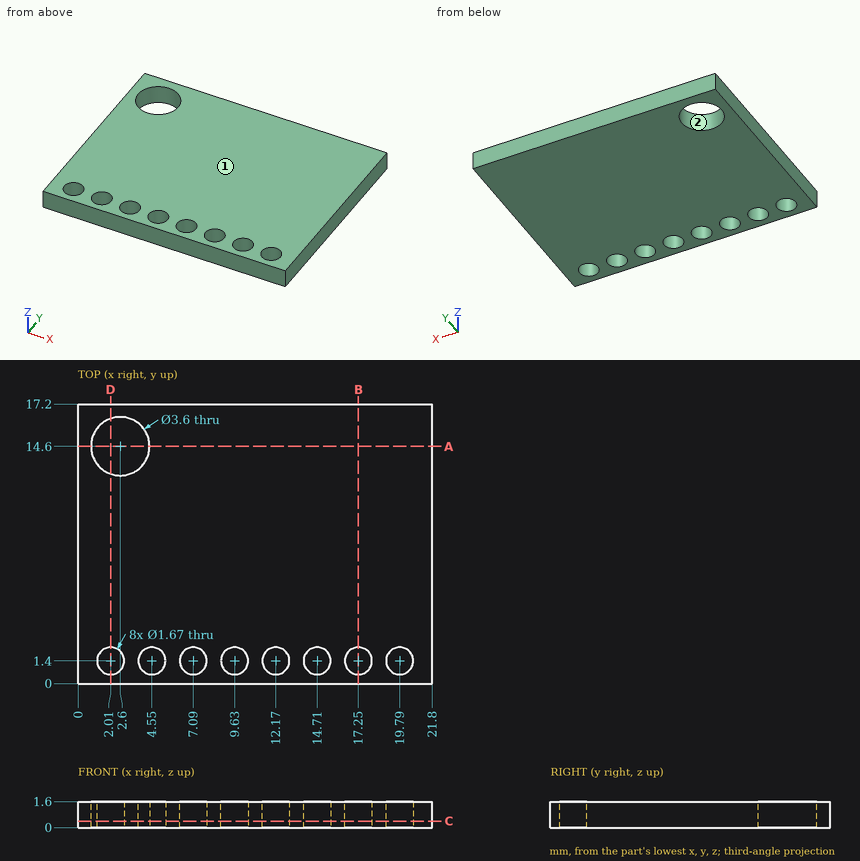
Source: three-view drawing plus pictorial views. Frame: mm from the lowest corner of the part. Round coordinates to 2 decimals unless told otherwise and drop trailing zeros. Loops run counter-clockwise (first coordinate to the right, second up) from the corner with the lowest first, then second, coordinate; pieces in that order, holes last.
1. Contact query for a flat-ended pin moving along its axis: pin 1 (6 mm diameter, centred on x = 10.5, y = 11.5, fed in from -Z). Output: stop coordinate, or through.
2. Section query C-C on z = 0.4. Give the number of separate pieces and of enclosed holes in the cut face, and give its area (3 significant figures).
3. Section query D-D on x = 2.01. Output: boundary loops of the cut face in (y, z) (3 decimals), and give its area (3 significant figures).
4. Section query B-B on x = 17.25. Output: boundary loops of the cut face in (y, z) (3 decimals).
5. Section query A-A on y = 14.6. Output: boundary loops of the cut face in (x, z), and give its area (3 significant figures).
6. Mould query, pull axis Y, two halves, no side actions, for the marked faces 1 and 2. Classes: released by +Y, released by -Y, zero draft, split by the parting line, or undercut.
7. Ray query, L1, parallel to Y at x = 19.79, z = 1.3 (3 decimals); L2, parallel to Y at x = 1.75, z = 0.3; L3, parallel to Y at x = 3.25, z = 0.9. Return the intervals inside material, ascending.
Answers below:
1. pin 1: stops at z = 0
2. separate pieces: 1
2. enclosed holes: 9
2. area: 347 mm2
3. outline: (0, 0) - (0.565, 0) - (0.565, 1.6) - (0, 1.6) - close; (2.235, 0) - (12.899, 0) - (12.899, 1.6) - (2.235, 1.6) - close; (16.301, 0) - (17.2, 0) - (17.2, 1.6) - (16.301, 1.6) - close
3. area: 19.4 mm2
4. outline: (0, 0) - (0.565, 0) - (0.565, 1.6) - (0, 1.6) - close; (2.235, 0) - (17.2, 0) - (17.2, 1.6) - (2.235, 1.6) - close
5. outline: (0, 0) - (0.8, 0) - (0.8, 1.6) - (0, 1.6) - close; (4.4, 0) - (21.8, 0) - (21.8, 1.6) - (4.4, 1.6) - close
5. area: 29.1 mm2
6. face 1: zero draft
6. face 2: undercut
7. L1: y = 0 to 0.565, 2.235 to 17.2
7. L2: y = 0 to 0.61, 2.19 to 13.01, 16.19 to 17.2
7. L3: y = 0 to 12.92, 16.28 to 17.2
